Read the model definition and answer for the solid it produces. Units are mm, in the model's axes. Face numbers are marked on the shaded views. A direction names the side the tool comes from. Round coordinates to 2 decimals unless told otherwise and drop trailing zeros. Order: outer loops, then holes, each group sorted by start corner. A loop starts at its lowest first (then second) coordinate and runs counter-clockwise, first axis right, second up. Notation, with made-up numbers: (57.5, -28) - (62.5, -28) arc R9 cw to (62.5, -17) - close; hole circle Ø2 at (65, -38). An arc over 180 degrees is marked (long way). Answer as a JSON object with one key per item and string values. Group by question number.
Q1. Consider line 1 (Y direction, x = -7, z = -20.25); line 2 (Y direction, x = 0, z = -20.8). Determine where each line is inside the solid, lowest interval first.
Q2. A tool of negligible diameter and unlimited length cuts with its end or side. For the marked faces 1, 2 and 3, from which of +Z, -Z, +X, -X, +Y, -Y can it reach the whole face along a straight path? Write none if from no direction.
Q3. Given pin 1 Ø1.1 at (x, z) = (-9.5, -25.5) entering from -Y; pin 2 Ø6 at (x, y) = (0, 0) entering from +Z; pin 3 Ø0.7 at (x, z) = (-9, -26.5) entering from +Y, each flat-ended and moving along its own axis, determine where each tip first touches the part or whether it passes through.
Q4. A cutting plane is placed at A-A on z = -18.5. Determine the outline of the cut face in (x, y), and give its area (3 significant figures).
Q5. A cutting plane is placed at B-B on z = -23.5. Determine the outline of the cut face in (x, y), and give its area (3 significant figures).
Q6. A cutting plane is placed at C-C on x = -8. Determine the outline of the cut face in (y, z), and give its area (3 significant figures).
Q7. The mould has two halves that part along X. Classify the marked faces 4, 5, 6 and 7: pulls with the +X half, pulls with the -X half, needs draft (parallel to the pull), parting line crosses it, or undercut.
```python
from build123d import *

# Parameters (mm, degrees)
BOSS_EXTRUDE1_DEPTH      = 23
BOSS_EXTRUDE1_2_DEPTH    = 23
SKETCH2_W                = 7
SKETCH2_H                = 7.5
CUT_EXTRUDE1_DEPTH       = 22
BOSS_EXTRUDE2_DEPTH      = 1.5
BOSS_EXTRUDE2_DEPTH_BACK = 0.5
FILLET1_R                = 0.5
SKETCH4_R                = 3.5
SKETCH4_R_2              = 2.5
BOSS_EXTRUDE3_DEPTH      = 5.5
SKETCH5_W                = 1.35
SKETCH5_H                = 6.2
BOSS_EXTRUDE4_DEPTH      = 5.5


with BuildPart() as part:
    # Sketch1 → Boss-Extrude1 (new body)
    with BuildSketch(Plane.XY):
        Polygon((-8.65, 8.65), (-1.4, 8.65), (-1.4, 10), (-10, 10), (-10, -10), (-1.4, -10), (-1.4, -8.65), (-8.65, -8.65), align=None)
    extrude(amount=-BOSS_EXTRUDE1_DEPTH)


with BuildPart() as body_2:
    # Sketch1 → Boss-Extrude1 2 (new body)
    with BuildSketch(Plane.XY):
        Polygon((10, -10), (10, 10), (1.4, 10), (1.4, 8.65), (8.65, 8.65), (8.65, -8.65), (1.4, -8.65), (1.4, -10), align=None)
    extrude(amount=-BOSS_EXTRUDE1_2_DEPTH)


with BuildPart() as cut_extrude1_tool:
    # Sketch2 → Cut-Extrude1 (new body)
    with BuildSketch(Plane.XZ.offset(10)):
        with Locations((0, -19.25)):
            Rectangle(SKETCH2_W, SKETCH2_H)
    extrude(amount=-CUT_EXTRUDE1_DEPTH)


with BuildPart() as part_1:
    add(part.part)

    # Cut-Extrude1: cut by cut_extrude1_tool
    add(cut_extrude1_tool.part, mode=Mode.SUBTRACT)



with BuildPart() as body_2_1:
    add(body_2.part)

    # Cut-Extrude1: cut by cut_extrude1_tool
    add(cut_extrude1_tool.part, mode=Mode.SUBTRACT)


with BuildPart() as part_2:
    add(part_1.part)

    add(body_2_1.part)  # Boss-Extrude2 merges body 2
    # Sketch3 → Boss-Extrude2 (add, two sides: drawn at the far end of the back side and taken through both)
    with BuildSketch(Plane(origin=(0, 0, -15.5), x_dir=(-1, 0, 0), z_dir=(0, 0, -1)).offset(-BOSS_EXTRUDE2_DEPTH_BACK)):
        Polygon((8.65, 8.65), (3.5, 8.65), (3.5, 5), (-3.5, 5), (-3.5, 8.65), (-8.65, 8.65), (-8.65, -8.65), (-3.5, -8.65), (-3.5, -5), (3.5, -5), (3.5, -8.65), (8.65, -8.65), align=None)
    extrude(amount=BOSS_EXTRUDE2_DEPTH + BOSS_EXTRUDE2_DEPTH_BACK)

    # Fillet1
    fillet1_edges = [part_2.edges().sort_by_distance(p)[0] for p in [
        (10, 10, -11.5),
        (10, -10, -11.5),
        (-10, -10, -11.5),
        (-10, 10, -11.5),
    ]]
    fillet(fillet1_edges, radius=FILLET1_R)

    # Sketch4 → Boss-Extrude3 (add)
    with BuildSketch(Plane(origin=(0, 0, -17), x_dir=(-1, 0, 0), z_dir=(0, 0, -1))):
        with Locations(Location((0, 0, 0), (0, 0, 180))):
            Circle(SKETCH4_R)
        Circle(SKETCH4_R_2, mode=Mode.SUBTRACT)
    extrude(amount=BOSS_EXTRUDE3_DEPTH)

    # Sketch5 → Boss-Extrude4 (add)
    with BuildSketch(Plane(origin=(0, 0, -23), x_dir=(-1, 0, 0), z_dir=(0, 0, -1))):
        with Locations((-9.325, 0)):
            Rectangle(SKETCH5_W, SKETCH5_H)
        with Locations((9.325, 0)):
            Rectangle(SKETCH5_W, SKETCH5_H)
    extrude(amount=BOSS_EXTRUDE4_DEPTH)


solid = part_2.part
```
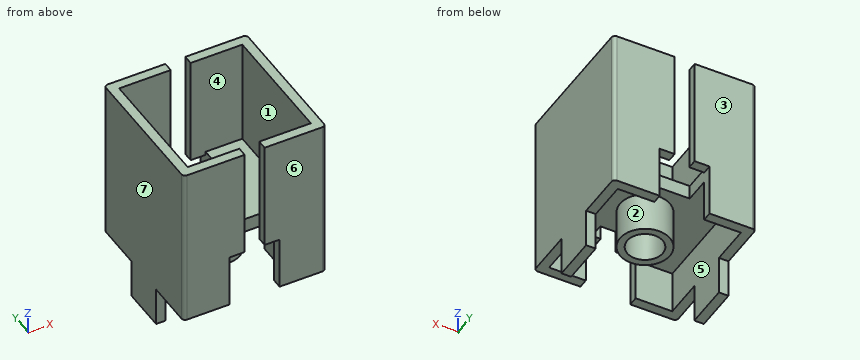
Result set:
{
 "1": {"line 1": "y = -10 to -8.65, 8.65 to 10", "line 2": "y = -3.5 to -2.5, 2.5 to 3.5"},
 "2": {"face 1": "+Z", "face 2": "-Z", "face 3": "+Z, -Z, +X, -X, +Y"},
 "3": {"pin 1": "stops at y = -3.1", "pin 2": "stops at z = -15", "pin 3": "stops at y = 3.1"},
 "4": {"outline": "(-10, -9.5) arc R0.5 ccw to (-9.5, -10) - (-3.5, -10) - (-3.5, -8.65) - (-8.65, -8.65) - (-8.65, 8.65) - (-3.5, 8.65) - (-3.5, 10) - (-9.5, 10) arc R0.5 ccw to (-10, 9.5) - close; circle Ø7 at (0, 0); (3.5, -10) - (9.5, -10) arc R0.5 ccw to (10, -9.5) - (10, 9.5) arc R0.5 ccw to (9.5, 10) - (3.5, 10) - (3.5, 8.65) - (8.65, 8.65) - (8.65, -8.65) - (3.5, -8.65) - close; hole circle Ø5 at (0, 0)", "area": "100 mm²"},
 "5": {"outline": "(-10, -3.1) - (-8.65, -3.1) - (-8.65, 3.1) - (-10, 3.1) - close; (8.65, -3.1) - (10, -3.1) - (10, 3.1) - (8.65, 3.1) - close", "area": "16.7 mm²"},
 "6": {"outline": "(-10, -23) - (-8.65, -23) - (-8.65, -17) - (8.65, -17) - (8.65, -23) - (10, -23) - (10, 0) - (8.65, 0) - (8.65, -15) - (-8.65, -15) - (-8.65, 0) - (-10, 0) - close", "area": "96.7 mm²"},
 "7": {"face 4": "undercut", "face 5": "undercut", "face 6": "needs draft", "face 7": "pulls with the -X half"}
}
